The model under review builds one solid part; all positions refer to its coordinate system, in mm. Coordinates: 2 decimals unless noted, no trailing zeros. Write each loop counter-clockwise with the first axis right and the second up, starting at its lowest first coordinate (ties: lowest second). Pieces come first, ordered by that corner, then holes. Notation, with made-up numbers: (44.25, 81.25) - (50.25, 81.25) arc R24 ccw to (50.25, 120.25) - close; hole circle Ø11 at (65, 19). An arc over 180 degrees is marked (long way). Put each result on its own line as item: value.
Autodesk Inventor part; units mm, degrees
ref_plane "YZ Plane" through (0, 0, 0) normal (1, 0, 0) x (0, 1, 0)
ref_plane "XZ Plane" through (0, 0, 0) normal (0, 1, 0) x (-1, 0, 0)
ref_plane "XY Plane" through (0, 0, 0) normal (0, 0, 1) x (1, 0, 0)
sketch "Sketch1" plane through (0, 0, 0) normal (0, 0, 1) x (1, 0, 0)
  circle A0 centre (0, 0) radius 19.05
  circle A1 centre (6.35, 6.35) radius 3.175
  circle A2 centre (-6.35, 6.35) radius 3.175
  circle A3 centre (-6.35, -6.35) radius 3.175
  circle A4 centre (6.35, -6.35) radius 3.175
  line L0 (0, 0) -> (0, 38.1233) construction
  line L1 (0, 0) -> (30.2858, 0) construction
  dimension "d0" = 38.1
  dimension "d1" = 6.35
  dimension "d4" = 360
  dimension "d6" = 6.35
  dimension "d7" = 6.35
extrude "Extrusion1" add sketch "Sketch1" along normal blind 6.35
properties part number "ShoulderBracketXZPlate"
1. Consider section A-A on x = 8.5. State the section outline as (y, z) points, plus the area to 3 significant figures.
Determined:
outline: (-17.05, 0) - (-8.69, 0) - (-8.69, 6.35) - (-17.05, 6.35) - close; (-4.01, 0) - (4.01, 0) - (4.01, 6.35) - (-4.01, 6.35) - close; (8.69, 0) - (17.05, 0) - (17.05, 6.35) - (8.69, 6.35) - close
area: 157 mm^2
2. Consider section C-C on z = 2.5. State the section outline as (x, y) points (3 decimals).
Determined:
outline: circle Ø38.1 at (0, 0); hole circle Ø6.35 at (-6.35, -6.35); hole circle Ø6.35 at (-6.35, 6.35); hole circle Ø6.35 at (6.35, -6.35); hole circle Ø6.35 at (6.35, 6.35)
3. Consider section B-B on y = 6.35. State the section outline as (x, z) points (3 decimals), plus the area to 3 significant figures.
Determined:
outline: (-17.961, 0) - (-9.525, 0) - (-9.525, 6.35) - (-17.961, 6.35) - close; (-3.175, 0) - (3.175, 0) - (3.175, 6.35) - (-3.175, 6.35) - close; (9.525, 0) - (17.961, 0) - (17.961, 6.35) - (9.525, 6.35) - close
area: 147 mm^2
4. The part is to be moulded in two halves that separate along Y. For faces 1 (the flat face through (0, 0, 0)), 2 (the cylindrical face through (3.83, 8.28, 3.13)), 3 (the cylindrical face through (-15.12, 11.59, 3.13)), 4 (the cylindrical face through (-7.04, 9.45, 3.13)), say which applies: +Y half, -Y half, draft (parallel to the pull), parting line (faces both ways), or undercut.
Determined:
face 1: draft
face 2: undercut
face 3: parting line
face 4: undercut
5. Consider section D-D on x = -15.5. State the section outline as (y, z) points, plus the area to 3 significant figures.
Determined:
outline: (-11.07, 0) - (11.07, 0) - (11.07, 6.35) - (-11.07, 6.35) - close
area: 141 mm^2
6. To check wall thickness, follow probe 1 along Y at (x, z) = (-6, 1); probe 2 along X at (y, z) = (-4.5, 0.5); probe 3 along Y at (x, z) = (-6.35, 3.25) (3 decimals). State the ranges of each line that lie inside material, in increasing order.
Determined:
probe 1: y = -18.08 to -9.51, -3.19 to 3.19, 9.51 to 18.08
probe 2: x = -18.51 to -8.93, -3.77 to 3.77, 8.93 to 18.51
probe 3: y = -17.961 to -9.525, -3.175 to 3.175, 9.525 to 17.961
7. For pin 1 Ø1 at (y, z) = (-4.5, 1) entering from -X, flat-tipped, find the tip position at first contact; note if it passes through.
Determined:
pin 1: stops at x = -18.63
